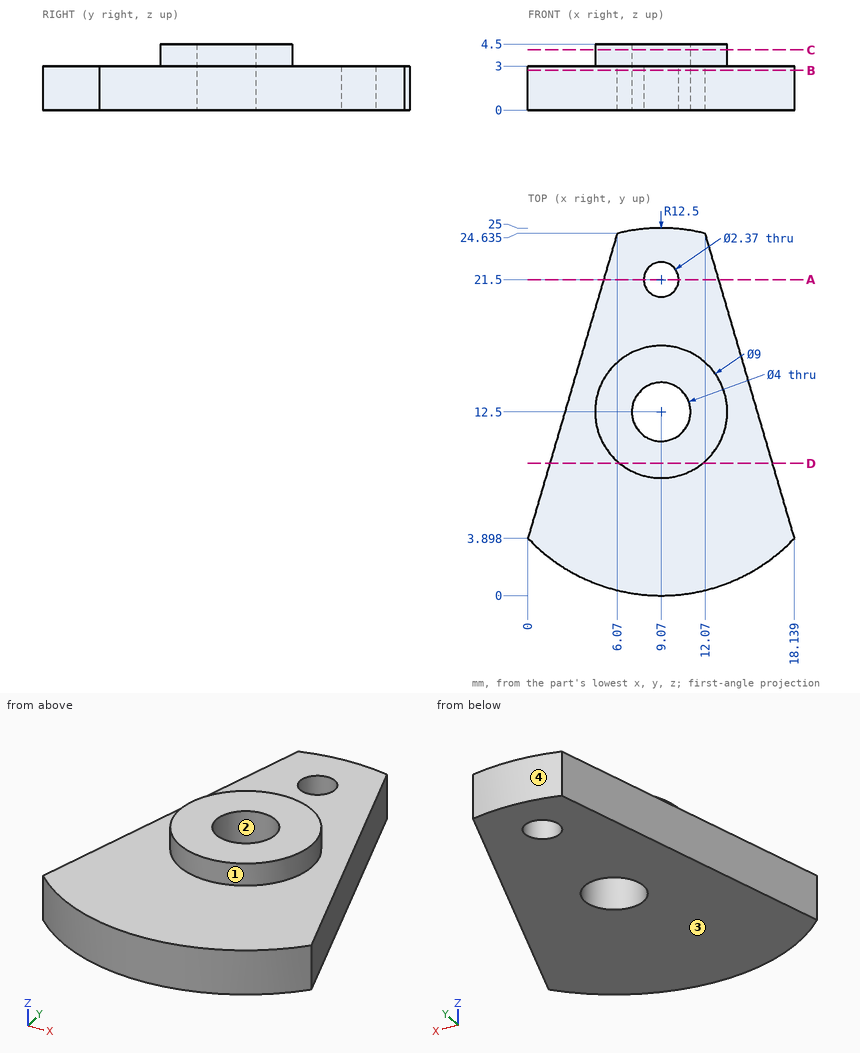
Here's the drawing with two shaded views (mm, measured from the low corner). I have some questions. Coordinates: 2 decimals unless noted, no trailing zeros. Loops run counter-clockwise (first coordinate to the right, second up) from the corner with the lowest first, then second, coordinate; pieces in that order, holes last. Notation, with made-up numbers: M -11,56.5 L 15,56.5 A14 cw 15,71.5 Z; hole C 35.5,82 d9. An arc over 180 degrees is marked long. Return JSON: item names as keys, results as strings. Group by question number.
Item 1: I'm going to push flat-ended pins straight in: pin 1 Ø1.5 at (y, z) = (7.5, 2) entering from +X (1 decimal); pin 2 Ø4 at (x, y) = (9.07, 21.5) entering from +Z; pin 3 Ø1 at (x, z) = (8, 1.5) entering from +Y; pin 4 Ø8 at (x, y) = (16, 8.5) entering from +Z. Where does each tip first touch, or does it pass through?
Item 2: Imagine slicing it at B-B (z = 2.7). Please give me the cut outline in (x, y) (1 decimal).
Item 3: Thinking about a two-plate mould opening in Y: for the marked faces 1, 2, 3 and 4, which applies, released by +Y, released by -Y, zero draft, split by the parting line, or undercut?
Item 4: Imagine slicing it at D-D (y = 9). Please give me the cut outline in (x, z).
Item 5: If I drill on L1, parallel to Z at x = 7, y = 18.25; L2, parallel to Y at x = 9.25, z = 3.55; L3, parallel to X at y = 14, z = 3.2 (1 decimal), over which ranges is the centre line in solid material (lowest first)? Write a range as from..to.
Item 6: Imagine slicing it at C-C (z = 4.1). Please give me the cut outline in (x, y).
Item 7: Imagine slicing it at A-A (y = 21.5). Please give me the cut outline in (x, z) (1 decimal), and give its area (3 significant figures).
Verdict:
{
 "1": {"pin 1": "stops at x = 17.3", "pin 2": "stops at z = 3", "pin 3": "stops at y = 24.99", "pin 4": "stops at z = 4.5"},
 "2": {"outline": "M 0,3.9 A12.5 ccw 18.1,3.9 L 12.1,24.6 A12.5 ccw 6.1,24.6 Z; hole C 9.1,12.5 d4; hole C 9.1,21.5 d2.4"},
 "3": {"face 1": "split by the parting line", "face 2": "undercut", "face 3": "zero draft", "face 4": "released by +Y"},
 "4": {"outline": "M 1.49,0 L 16.65,0 L 16.65,3 L 11.9,3 L 11.9,4.5 L 6.24,4.5 L 6.24,3 L 1.49,3 Z"},
 "5": {"L1": "z = 0..3", "L2": "y = 8..10.51, 14.49..17", "L3": "x = 4.8..7.7, 10.4..13.3"},
 "6": {"outline": "C 9.07,12.5 d9; hole C 9.07,12.5 d4"},
 "7": {"outline": "M 5.2,0 L 7.9,0 L 7.9,3 L 5.2,3 Z; M 10.3,0 L 13,0 L 13,3 L 10.3,3 Z", "area": "16.4 mm^2"}
}
